Geometry: final body of the model. Coordinates: model frame, mm. Give positions to 0.01 mm unless a question says otherwise; leave off trailing zeros. Loops run counter-clockwise (first coordinate to the right, second up) from the corner with the lowest first, then second, coordinate; pieces in that order, holes last. Notation, with made-up numbers: (-30, 6.5) -> (-6, 6.5) arc R36 cw to (-6, 45.5) -> close; hole circle Ø2 at (4, -20). An arc over 180 degrees is marked (long way). Answer in a Markdown table with one row per item. Add a question column.
1) Section query D-D (x = 7.5). Return the cut outline in (y, z), plus the area to 3 significant figures.
2) Section query A-A (x = 32.5). Return the cut outline in (y, z), plus the area to 3 significant figures.
3) First-contact query: P1, Ø3, axis at y = 3, z = -67, coming from the -X side. Flat tip, straight axial feed; report the tip coordinate or a pass-through.
4) Section query C-C (y = 3.4). Give the number of separate pieces and of enclosed holes in the cut face, plus the area to 3 significant figures.
5) Section query B-B (z = -84.5). Return the cut outline in (x, y).
6) Line query: line 1 (Z direction, x = 4, y = 4.6); line 2 (X direction, y = 3.25, z = -18); line 3 (Z direction, x = 8.5, y = 2.4). Output: solid intervals per line, ascending. Write a range as from..to.
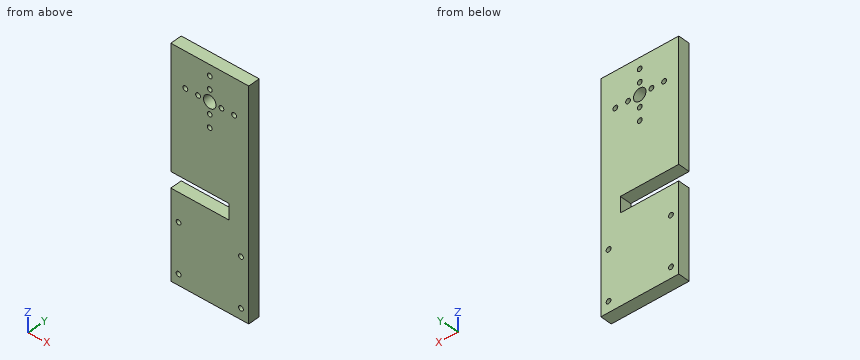
Autodesk Inventor part; units mm, degrees
ref_plane "YZ Plane" through (0, 0, 0) normal (1, 0, 0) x (0, 1, 0)
ref_plane "XZ Plane" through (0, 0, 0) normal (0, 1, 0) x (-1, 0, 0)
ref_plane "XY Plane" through (0, 0, 0) normal (0, 0, 1) x (1, 0, 0)
sketch "スケッチ1" plane through (0, 0, 0) normal (0, 1, 0) x (-1, 0, 0)
  line L0 (0, 0) -> (-40, 0)
  line L1 (-40, 0) -> (-40, -115)
  line L2 (-40, -115) -> (0, -115)
  line L3 (0, -115) -> (0, 0)
  dimension "d0" = 40
  dimension "d1" = 115
extrude "押し出し1" add sketch "スケッチ1" along normal blind 6
sketch "スケッチ2" plane through (0, 6, 0) normal (0, 1, 0) x (1, 0, 0)
  line L0 (0, 0) -> (40, 0) construction
  line L1 (20, 0) -> (20, 115) construction
  line L2 (40, 115) -> (0, 115) construction
  point P0 (20, 18)
  dimension "d4" = 18
hole "穴1" at (20, 6, -18) direction (0, -1, 0) diameter 6.4 end through all
sketch "スケッチ3" plane through (0, 6, 0) normal (0, 1, 0) x (1, 0, 0)
  circle A0 centre (20, 18) radius 3.2 construction
  circle A1 centre (20, 18) radius 12.5 construction
  point P0 (0, 0)
  point P1 (7.5, 18)
  point P2 (20, 5.5)
  point P3 (32.5, 18)
  point P4 (20, 30.5)
  dimension "d12" = 25
  dimension "d15" = 360
hole "穴2" at (7.5, 6, -18) at (20, 6, -5.5) at (32.5, 6, -18) at (20, 6, -30.5) direction (0, -1, 0) diameter 2.459 end through all
sketch "スケッチ4" plane through (0, 6, 0) normal (0, 1, 0) x (1, 0, 0)
  line L0 (40, 115) -> (0, 115) construction
  line L1 (0, 115) -> (40, 115) construction
  line L2 (40, 115) -> (40, 110) construction
  line L3 (40, 110) -> (0, 110) construction
  line L4 (0, 110) -> (0, 115) construction
  line L5 (0, 115) -> (0, 0)
  line L6 (0, 112.5) -> (40, 112.5) construction
  line L7 (40, 0) -> (40, 115)
  line L8 (0, 115) -> (0, 0) construction
  line L9 (40, 85) -> (0, 85) construction
  line L10 (0, 85) -> (0, 90) construction
  line L11 (0, 90) -> (40, 90) construction
  line L12 (40, 90) -> (40, 85) construction
  line L13 (40, 87.5) -> (0, 87.5) construction
  point P0 (4, 112.5)
  point P1 (36, 112.5)
  point P2 (36, 87.5)
  point P3 (4, 87.5)
  dimension "d25" = 5
  dimension "d26" = 4
  dimension "d27" = 4
  dimension "d35" = 5
  dimension "d36" = 25
hole "穴3" [suppressed]
sketch "スケッチ5" plane through (0, 0, 0) normal (0, -1, 0) x (1, 0, 0)
  line L0 (30, -62) -> (0, -62)
  line L1 (0, -62) -> (0, -70)
  line L2 (0, -70) -> (30, -70)
  line L3 (30, -70) -> (30, -62)
  line L4 (0, 0) -> (40, 0)
  dimension "d37" = 8
  dimension "d38" = 62
  dimension "d39" = 30
extrude "押し出し2" cut sketch "スケッチ5" against normal blind 10
sketch "スケッチ6" plane through (0, 6, 0) normal (0, 1, 0) x (1, 0, 0)
  line L0 (36, 84.5) -> (4, 84.5) construction
  line L1 (4, 84.5) -> (4, 109.5) construction
  line L2 (4, 109.5) -> (36, 109.5) construction
  line L3 (36, 109.5) -> (36, 84.5) construction
  line L4 (40, 0) -> (40, 115) construction
  line L5 (0, 115) -> (0, 70) construction
  line L6 (40, 115) -> (0, 115) construction
  point P0 (0, 0)
  point P1 (20, 109.5)
  dimension "d42" = 4
  dimension "d43" = 4
  dimension "d44" = 5.5
  dimension "d45" = 25
hole "穴4" at (36, 6, -84.5) at (36, 6, -109.5) at (4, 6, -109.5) at (4, 6, -84.5) direction (0, -1, 0) diameter 2.459 end through all
sketch "スケッチ7" plane through (0, 6, 0) normal (0, 1, 0) x (1, 0, 0)
  circle A0 centre (20, 18) radius 3.2
  circle A1 centre (20, 18) radius 6
  point P0 (0, 0)
  point P1 (20, 12)
  point P2 (14, 18)
  point P3 (20, 24)
  point P4 (26, 18)
  dimension "d53" = 12
hole "穴5" at (20, 6, -12) at (14, 6, -18) at (20, 6, -24) at (26, 6, -18) direction (0, -1, 0) diameter 2.459 end through all
properties part number "shoulder1_lower_cover" material "アルミニウム 5052"
Evaluation:
| question | item | result |
|---|---|---|
| 1 | outline | (0, -115) -> (6, -115) -> (6, -70) -> (0, -70) -> close; (0, -62) -> (6, -62) -> (6, -19.23) -> (0, -19.23) -> close; (0, -16.77) -> (6, -16.77) -> (6, 0) -> (0, 0) -> close |
| 1 | area | 627 mm² |
| 2 | outline | (0, -115) -> (6, -115) -> (6, -19.23) -> (0, -19.23) -> close; (0, -16.77) -> (6, -16.77) -> (6, 0) -> (0, 0) -> close |
| 2 | area | 675 mm² |
| 3 | P1 | x = 30 |
| 4 | separate pieces | 1 |
| 4 | enclosed holes | 13 |
| 4 | area | 4,270 mm² |
| 5 | outline | (0, 0) -> (2.77, 0) -> (2.77, 6) -> (0, 6) -> close; (5.23, 0) -> (34.77, 0) -> (34.77, 6) -> (5.23, 6) -> close; (37.23, 0) -> (40, 0) -> (40, 6) -> (37.23, 6) -> close |
| 6 | line 1 | -115..-110.73, -108.27..-85.73, -83.27..-70, -62..0 |
| 6 | line 2 | 0..6.27, 8.73..12.77, 15.23..16.8, 23.2..24.77, 27.23..31.27, 33.73..40 |
| 6 | line 3 | -115..-70, -62..-18.72, -17.28..0 |
